Work out the finished part from the listing and answer in its coordinate system (mm). Give positions to 0.01 mm unless a question says otherwise; leave off trailing zeros. Loops run counter-clockwise (first coordinate to the right, second up) from the corner with the lowest first, then second, coordinate; pieces in that order, holes last. Notation, with made-up numbers: (68.25, 44) - (111.25, 44) arc R30 cw to (111.25, 67) - close; hole circle Ø5 at (73, 17.25). An arc over 180 degrees is marked (long way). Use CSV: the item, a comma, the result in double quotes.
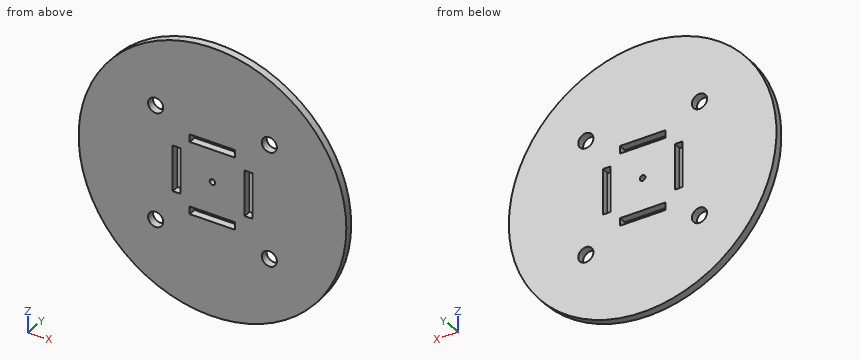
from build123d import *

# Parameters (mm, degrees)
SKETCH1_R           = 53
BOSS_EXTRUDE1_DEPTH = 3
SKETCH2_R           = 1.1
SKETCH2_W           = 18
SKETCH2_H           = 3
SKETCH2_W_2         = 3
SKETCH2_H_2         = 18
CUT_EXTRUDE1_DEPTH  = 3
SKETCH4_R           = 3
CUT_EXTRUDE2_DEPTH  = 3
CIRPATTERN1_COUNT   = 4


with BuildPart() as part:
    # Sketch1 → Boss-Extrude1 (new body)
    with BuildSketch(Plane(origin=(0, 0, 0), x_dir=(1, 0, 0), z_dir=(0, 1, 0))):
        Circle(SKETCH1_R)
    extrude(amount=BOSS_EXTRUDE1_DEPTH)

    # Sketch2 → Cut-Extrude1 (cut)
    with BuildSketch(Plane(origin=(0, 3, 0), x_dir=(1, 0, 0), z_dir=(0, 1, 0))):
        Circle(SKETCH2_R)
        with Locations((0, 14.25)):
            Rectangle(SKETCH2_W, SKETCH2_H)
        with Locations((-14.25, 0)):
            Rectangle(SKETCH2_W_2, SKETCH2_H_2)
        with Locations((0, -14.25)):
            Rectangle(SKETCH2_W, SKETCH2_H)
        with Locations((14.25, 0)):
            Rectangle(SKETCH2_W_2, SKETCH2_H_2)
    extrude(amount=-CUT_EXTRUDE1_DEPTH, mode=Mode.SUBTRACT)

    # Sketch4 → Cut-Extrude2 (cut)
    with BuildSketch(Plane(origin=(0, 3, 0), x_dir=(1, 0, 0), z_dir=(0, 1, 0))):
        with Locations((-22.5, 22.5)):
            Circle(SKETCH4_R)
    cut_extrude2 = extrude(amount=-CUT_EXTRUDE2_DEPTH, mode=Mode.SUBTRACT)

    # CirPattern1: Cut-Extrude2 ×4 about axis
    cirpattern1_axis = Axis((0, 0, 0), (0, 1, 0))
    for i in range(1, CIRPATTERN1_COUNT):
        add(cut_extrude2.rotate(cirpattern1_axis, i * 360 / CIRPATTERN1_COUNT), mode=Mode.SUBTRACT)


solid = part.part
Item 1: A cutting plane is placed at B-B on y = 1.4. State how many separate pieces and enclosed holes the cut face has, and give its area (3 significant figures).
Determined:
separate pieces,"1"
enclosed holes,"9"
area,"8,490 mm²"
Item 2: A cutting plane is placed at D-D on z = 11. Determine the outline of the cut face in (x, y).
Determined:
outline,"(-51.85, 0) - (51.85, 0) - (51.85, 3) - (-51.85, 3) - close"
Item 3: Find the intervals of material crossed by line 1 (Z direction, x = 0, y = 1.1); line 2 (X direction, y = 1.6, z = -22.5), in increasing order.
Determined:
line 1,"z = -53 to -15.75, -12.75 to -1.1, 1.1 to 12.75, 15.75 to 53"
line 2,"x = -47.99 to -25.5, -19.5 to 19.5, 25.5 to 47.99"
Item 4: A cutting plane is placed at A-A on z = -22.5. Determine the outline of the cut face in (x, y), and give its area (3 significant figures).
Determined:
outline,"(-47.99, 0) - (-25.5, 0) - (-25.5, 3) - (-47.99, 3) - close; (-19.5, 0) - (19.5, 0) - (19.5, 3) - (-19.5, 3) - close; (25.5, 0) - (47.99, 0) - (47.99, 3) - (25.5, 3) - close"
area,"252 mm²"
Item 5: Given P1, Ø1, axis at x = -24.5, y = 1.5, coming from the -Z side; P2, Ø1, axis at x = 28, y = 1.5, coming from the -Z side; P3, Ø1.5, axis at x = 2, y = 2, coming from the -Z side; P4, Ø3.5, axis at x = 22.5, z = 22.5, coming from the -Y side, each flat-ended and moving along its own axis, determine where each tip first touches the part or whether it passes through.
Determined:
P1,"stops at z = -47.25"
P2,"stops at z = -45.31"
P3,"stops at z = -52.99"
P4,"passes through"
Item 6: A cutting plane is placed at C-C on x = -22.5. Determine the outline of the cut face in (y, z).
Determined:
outline,"(0, -47.99) - (3, -47.99) - (3, -25.5) - (0, -25.5) - close; (0, -19.5) - (3, -19.5) - (3, 19.5) - (0, 19.5) - close; (0, 25.5) - (3, 25.5) - (3, 47.99) - (0, 47.99) - close"
